Check sheet for the modelled part. Datum: model origin and axes. Units: mm. Face numbers are marked on the shaded views. A direction names the side the tool comes from. Round coordinates to 2 decimals unless told otherwise and drop trailing zeros. Loops run counter-clockwise (first coordinate to the right, second up) from the corner with the lowest first, then second, coordinate; pieces in that order, holes last. Notation, with made-up numbers: (79.25, 43.5) - (93.25, 43.5) arc R33 ccw to (93.25, 79.5) - close; hole circle Ø3 at (-27.5, 12). An arc over 180 degrees is marked (long way). Answer in a Markdown table with one row per item. Add a question column.
(1) Cross-section at A-A on z = 17.5. Enter the section's corners in (x, y).
(2) Gauge pin test, flat ends, axial feed: pin 1 (8 mm diameter, centred on x = 17, z = -3, fed in from +Y); pin 2 (5 mm diameter, centred on y = -8.5, z = 15.5, fed in from +X); pin 3 (7.5 mm diameter, centred on x = 16.5, y = -4.5, fed in from -Z); pin 4 (1.5 mm diameter, centred on x = -3, y = -4, fed in from +Z). Record the tip position at first contact, or that the pin passes through.
(3) Cross-section at C-C on x = -25. Enter the section's corners in (y, z).
(4) Thickness scan on line 1 along Z through (x, y) = (-25.7, -7.5); line 2 along Z through (x, y) = (-21, -7.5); line 3 along X through (y, z) = (-12, 21). Record the ranges inside material, lowest first.
(5) Access from +Z, -Z, +X, -X, +Y, -Y to the whole of each face (thin tool, end or side, straight path). Record for the marked faces 1, 2, 3 and 4.
(6) Cross-section at B-B on y = -7.5. Enter the section's corners in (x, z), then the cut area to 3 significant figures.
(7) Cross-section at D-D on y = -1. Enter the section's corners in (x, z), then the cut area to 3 significant figures.
(8) Mould release check, pull along Z, two halves, no side actions. Record for the marked faces 5, 6 and 7: +Z half, -Z half, draft (parallel to the pull), parting line (faces both ways), or undercut.
from build123d import *

# Parameters (mm, degrees)
F0_W     = 10
F0_H     = 15
F0_H_2   = 20
F1_DEPTH = 15
F2_R     = 3
F3_DEPTH = 10.001
F4_R     = 5
F4_R_2   = 3
F5_DEPTH = 4
F6_R     = 3
F7_DEPTH = 10.001
F8_R     = 5
F8_R_2   = 3
F9_DEPTH = 4


with BuildPart() as f1:
    # F0 (on Front) → F1 (new body)
    with BuildSketch(Plane.XZ):
        with Locations((-25, 17.5)):
            Rectangle(F0_W, F0_H)
        with Locations((-25, 0)):
            Rectangle(F0_W, F0_H_2)
        with BuildLine():
            Line((-20, -10), (30, -10))
            Line((30, -10), (30, 10))
            Line((30, 10), (25, 10))
            ThreePointArc((25, 10), (10, -5), (-5, 10))
            Line((-5, 10), (-20, 10))
            Line((-20, 10), (-20, -10))
        make_face()
        with Locations((-25, -17.5)):
            Rectangle(F0_W, F0_H)
    extrude(amount=F1_DEPTH)

    # F2 (on face) → F3 (cut, through all)
    with BuildSketch(Plane.YZ.offset(-20)):
        with Locations((-7.5, 17.5)):
            Circle(F2_R)
    extrude(amount=-F3_DEPTH, mode=Mode.SUBTRACT)

    # F4 (on face) → F5 (cut)
    with BuildSketch(Plane.YZ.offset(-20)):
        with Locations((-7.5, 17.5)):
            Circle(F4_R)
        with Locations((-7.5, 17.5)):
            Circle(F4_R_2, mode=Mode.SUBTRACT)
    extrude(amount=-F5_DEPTH, mode=Mode.SUBTRACT)

    # F6 (on face) → F7 (cut, through all)
    with BuildSketch(Plane.YZ.offset(-20)):
        with Locations((-7.5, -17.5)):
            Circle(F6_R)
    extrude(amount=-F7_DEPTH, mode=Mode.SUBTRACT)

    # F8 (on face) → F9 (cut)
    with BuildSketch(Plane.YZ.offset(-20)):
        with Locations((-7.5, -17.5)):
            Circle(F8_R)
        with Locations((-7.5, -17.5)):
            Circle(F8_R_2, mode=Mode.SUBTRACT)
    extrude(amount=-F9_DEPTH, mode=Mode.SUBTRACT)


solid = f1.part
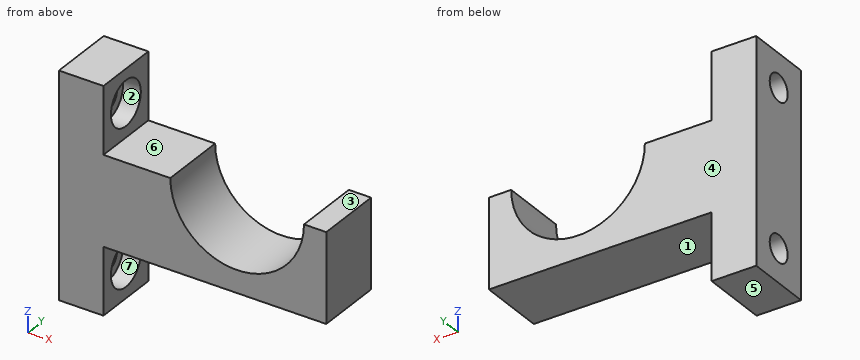
Answers:
| question | item | result |
|---|---|---|
| 1 | outline | (-30, -15) - (-20, -15) - (-20, -12.5) - (-24, -12.5) - (-24, -10.5) - (-30, -10.5) - close; (-30, -4.5) - (-24, -4.5) - (-24, -2.5) - (-20, -2.5) - (-20, 0) - (-30, 0) - close |
| 2 | pin 1 | stops at y = 0 |
| 2 | pin 2 | stops at x = -24 |
| 2 | pin 3 | stops at z = -10 |
| 2 | pin 4 | stops at z = 4.01 |
| 3 | outline | (-15, -25) - (0, -25) - (0, 25) - (-15, 25) - close; hole circle Ø6 at (-7.5, -17.5); hole circle Ø6 at (-7.5, 17.5) |
| 4 | line 1 | z = -25 to -20.5, -14.5 to 14.5, 20.5 to 25 |
| 4 | line 2 | z = -25 to -22.5, -12.5 to 12.5, 22.5 to 25 |
| 4 | line 3 | x = -30 to -20 |
| 5 | face 1 | -Z, +X, +Y, -Y |
| 5 | face 2 | +X |
| 5 | face 3 | +Z, +X, +Y, -Y |
| 5 | face 4 | +Z, -Z, +X, -X, +Y |
| 6 | outline | (-30, -25) - (-20, -25) - (-20, -22.5) - (-24, -22.5) - (-24, -20.5) - (-30, -20.5) - close; (-30, -14.5) - (-24, -14.5) - (-24, -12.5) - (-20, -12.5) - (-20, -10) - (30, -10) - (30, 10) - (25, 10) arc R15 cw to (-5, 10) - (-20, 10) - (-20, 12.5) - (-24, 12.5) - (-24, 14.5) - (-30, 14.5) - close; (-30, 20.5) - (-24, 20.5) - (-24, 22.5) - (-20, 22.5) - (-20, 25) - (-30, 25) - close |
| 6 | area | 995 mm^2 |
| 7 | outline | (-30, -25) - (-20, -25) - (-20, -10) - (30, -10) - (30, 10) - (25, 10) arc R15 cw to (-5, 10) - (-20, 10) - (-20, 25) - (-30, 25) - close |
| 7 | area | 1,150 mm^2 |
| 8 | face 5 | -Z half |
| 8 | face 6 | +Z half |
| 8 | face 7 | undercut |
